from build123d import *

# Parameters (mm, degrees)
SKETCH6_W            = 40
SKETCH6_H            = 30
BOSS_EXTRUDE1_DEPTH  = 6
SKETCH10_W           = 7
SKETCH10_H           = 7
CUT_EXTRUDE6_DEPTH   = 51.358713248
LPATTERN3_COUNT      = 3
LPATTERN3_PITCH      = 10
LPATTERN3_COUNT_DIR2 = 4
LPATTERN3_PITCH_DIR2 = 10
SKETCH11_W           = 3
SKETCH11_H           = 30
CUT_EXTRUDE7_DEPTH   = 3
LPATTERN4_COUNT      = 3
LPATTERN4_PITCH      = 10
SKETCH12_W           = 1.5
SKETCH12_H           = 30
CUT_EXTRUDE8_DEPTH   = 51.358713248


with BuildPart() as part:
    # Sketch6 → Boss-Extrude1 (new body)
    with BuildSketch(Plane(origin=(0, 0, 0), x_dir=(1, 0, 0), z_dir=(0, 1, 0))):
        with Locations((20, -15)):
            Rectangle(SKETCH6_W, SKETCH6_H)
    extrude(amount=BOSS_EXTRUDE1_DEPTH)

    # Sketch10 → Cut-Extrude6 (cut, through all)
    with BuildSketch(Plane(origin=(0, 6, 0), x_dir=(1, 0, 0), z_dir=(0, 1, 0))):
        with Locations((5, -5)):
            Rectangle(SKETCH10_W, SKETCH10_H)
    cut_extrude6 = extrude(amount=-CUT_EXTRUDE6_DEPTH, mode=Mode.SUBTRACT)

    # LPattern3: Cut-Extrude6 3 × 4
    with Locations(*[(j * LPATTERN3_PITCH_DIR2, 0, i * LPATTERN3_PITCH) for i in range(LPATTERN3_COUNT) for j in range(LPATTERN3_COUNT_DIR2) if (i, j) != (0, 0)]):
        add(cut_extrude6, mode=Mode.SUBTRACT)

    # Sketch11 → Cut-Extrude7 (cut)
    with BuildSketch(Plane(origin=(0, 6, 0), x_dir=(1, 0, 0), z_dir=(0, 1, 0))):
        with Locations((10, -15)):
            Rectangle(SKETCH11_W, SKETCH11_H)
    cut_extrude7 = extrude(amount=-CUT_EXTRUDE7_DEPTH, mode=Mode.SUBTRACT)

    # LPattern4: Cut-Extrude7 ×3
    with Locations(*[(i * LPATTERN4_PITCH, 0, 0) for i in range(1, LPATTERN4_COUNT)]):
        add(cut_extrude7, mode=Mode.SUBTRACT)

    # Sketch12 → Cut-Extrude8 (cut, through all)
    with BuildSketch(Plane(origin=(0, 6, 0), x_dir=(1, 0, 0), z_dir=(0, 1, 0))):
        with Locations((0.75, -15)):
            Rectangle(SKETCH12_W, SKETCH12_H)
        with Locations((39.25, -15)):
            Rectangle(SKETCH12_W, SKETCH12_H)
    extrude(amount=-CUT_EXTRUDE8_DEPTH, mode=Mode.SUBTRACT)


solid = part.part
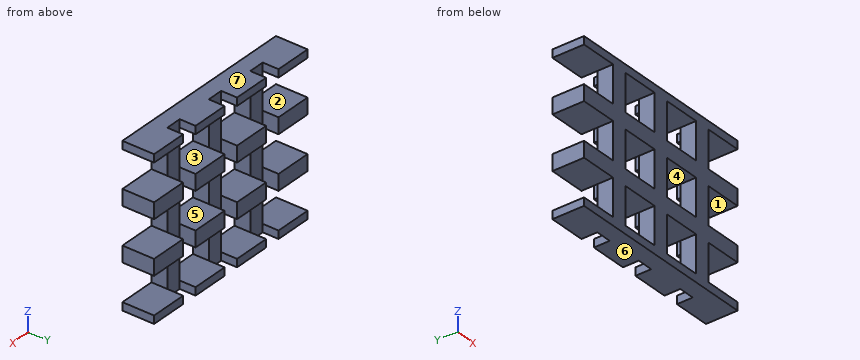
Could you check a few things on this model? Use its own coordinates, in mm. Face numbers are marked on the shaded views. A direction names the side the tool comes from. Coordinates: 2 decimals unless noted, no trailing zeros. Write each loop counter-clockwise with the first axis right and the second up, starting at its lowest first coordinate (ties: lowest second). Pieces come first, ordered by that corner, then holes. Notation, with made-up numbers: (71.25, 64) - (123.25, 64) arc R24 cw to (123.25, 92) - close; hole circle Ø5 at (-1, 15). An arc over 180 degrees is marked (long way). Write item = value, one per line.
1) Suppose I cut it at C-C on y = 5.2. State how many separate pieces and enclosed holes the cut face has, plus the area to 3 significant figures.
Result set:
separate_pieces = 16
enclosed_holes = 0
area = 252 mm2
2) We'd pull the mould along Z, two halves only. Please class the marked faces 4, 5, 6 and 7: +Z half, -Z half, draft (parallel to the pull), parting line (faces both ways), or undercut.
Result set:
face_4 = undercut
face_5 = undercut
face_6 = -Z half
face_7 = +Z half
3) Suppose I cut it at A-A on z = 3. Please give me the cut outline in (x, y), plus the area to 3 significant figures.
Result set:
outline = (8.5, 0) - (11.5, 0) - (11.5, 3) - (8.5, 3) - close; (18.5, 0) - (21.5, 0) - (21.5, 3) - (18.5, 3) - close; (28.5, 0) - (31.5, 0) - (31.5, 3) - (28.5, 3) - close
area = 27.0 mm2
4) Suppose I cut it at B-B on x = 6. Please give me the cut outline in (y, z).
Result set:
outline = (0, 0) - (6, 0) - (6, 1.5) - (0, 1.5) - close; (0, 8.5) - (6, 8.5) - (6, 11.5) - (0, 11.5) - close; (0, 18.5) - (6, 18.5) - (6, 21.5) - (0, 21.5) - close; (0, 28.5) - (6, 28.5) - (6, 30) - (0, 30) - close
5) For the marked faces 1, 2 and 3, which set-ups out of +Z, -Z, +X, -X, +Y, -Y let a thin tool reach every point of the face, with its end or its side?
Result set:
face_1 = +X, +Y, -Y
face_2 = -X, +Y, -Y
face_3 = +Y, -Y
6) Will these pins go through, and if not, where does the flat tip stop? pin 1 Ø1.5 at (x, z) = (20, 22) entering from +Y; pin 2 Ø3.5 at (y, z) = (1.5, 5) entering from -X; pin 3 Ø1.5 at (y, z) = (1.5, 14) entering from +X.
Result set:
pin_1 = 3
pin_2 = 8.5
pin_3 = 31.5
7) Please list where these lines run through material, in increasing order: line 1 (Z direction, x = 33.5, y = 2.35); line 2 (X direction, y = 3.5, z = 9); line 3 (X direction, y = 1.8, z = 14.75). Write a range as [from, to].
Result set:
line_1 = [0, 1.5], [8.5, 11.5], [18.5, 21.5], [28.5, 30]
line_2 = [1.5, 8.5], [11.5, 18.5], [21.5, 28.5], [31.5, 38.5]
line_3 = [8.5, 11.5], [18.5, 21.5], [28.5, 31.5]
